```python
from build123d import *

# Parameters (mm, degrees)
F0_R     = 9.525
F0_R_2   = 63.5
F0_R_3   = 31.75
F0_R_4   = 19.05
F0_R_5   = 6.35
F1_DEPTH = 19.05
F2_DEPTH = 76.2
F3_DEPTH = 50.8
F4_DEPTH = 38.1


with BuildPart() as f1:
    # F0 (on Top) → F1 (new body)
    with BuildSketch(Plane.XY):
        with BuildLine():
            ThreePointArc((0, 76.2), (53.881537, 53.881537), (76.2, 0))
            Line((76.2, 0), (88.9, 0))
            Line((88.9, 0), (88.9, 38.1))
            Line((88.9, 38.1), (107.95, 38.1))
            ThreePointArc((107.95, 38.1), (127, 57.15), (107.95, 76.2))
            Line((107.95, 76.2), (0, 76.2))
        make_face()
        with Locations((107.95, 57.15)):
            Circle(F0_R, mode=Mode.SUBTRACT)
        with BuildLine():
            ThreePointArc((-76.2, 0), (-53.881537, 53.881537), (0, 76.2))
            Line((0, 76.2), (-107.95, 76.2))
            ThreePointArc((-107.95, 76.2), (-127, 57.15), (-107.95, 38.1))
            Line((-107.95, 38.1), (-88.9, 38.1))
            Line((-88.9, 38.1), (-88.9, 0))
            Line((-88.9, 0), (-76.2, 0))
        make_face()
        with Locations((-107.95, 57.15)):
            Circle(F0_R, mode=Mode.SUBTRACT)
        with BuildLine():
            Line((-107.95, -76.2), (0, -76.2))
            ThreePointArc((0, -76.2), (-53.881537, -53.881537), (-76.2, 0))
            Line((-76.2, 0), (-88.9, 0))
            Line((-88.9, 0), (-88.9, -38.1))
            Line((-88.9, -38.1), (-107.95, -38.1))
            ThreePointArc((-107.95, -38.1), (-127, -57.15), (-107.95, -76.2))
        make_face()
        with Locations((-107.95, -57.15)):
            Circle(F0_R, mode=Mode.SUBTRACT)
        with BuildLine():
            Line((88.9, 0), (76.2, 0))
            ThreePointArc((76.2, 0), (53.881537, -53.881537), (0, -76.2))
            Line((0, -76.2), (107.95, -76.2))
            ThreePointArc((107.95, -76.2), (127, -57.15), (107.95, -38.1))
            Line((107.95, -38.1), (88.9, -38.1))
            Line((88.9, -38.1), (88.9, 0))
        make_face()
        with Locations((107.95, -57.15)):
            Circle(F0_R, mode=Mode.SUBTRACT)
        with BuildLine():
            ThreePointArc((0, -76.2), (53.881537, -53.881537), (76.2, 0))
            ThreePointArc((76.2, 0), (53.881537, 53.881537), (0, 76.2))
            ThreePointArc((0, 76.2), (-53.881537, 53.881537), (-76.2, 0))
            ThreePointArc((-76.2, 0), (-53.881537, -53.881537), (0, -76.2))
        make_face()
        Circle(F0_R_2, mode=Mode.SUBTRACT)
        Circle(F0_R_2)
        Circle(F0_R_3, mode=Mode.SUBTRACT)
        Circle(F0_R_3)
        Circle(F0_R_4, mode=Mode.SUBTRACT)
        Circle(F0_R_4)
        Circle(F0_R_5, mode=Mode.SUBTRACT)
        Circle(F0_R_5)
    extrude(amount=F1_DEPTH)

    # F0 (on Top) → F2 (join)
    with BuildSketch(Plane.XY):
        with BuildLine():
            ThreePointArc((0, -76.2), (53.881537, -53.881537), (76.2, 0))
            ThreePointArc((76.2, 0), (53.881537, 53.881537), (0, 76.2))
            ThreePointArc((0, 76.2), (-53.881537, 53.881537), (-76.2, 0))
            ThreePointArc((-76.2, 0), (-53.881537, -53.881537), (0, -76.2))
        make_face()
        Circle(F0_R_2, mode=Mode.SUBTRACT)
    extrude(amount=F2_DEPTH)

    # F0 (on Top) → F3 (join)
    with BuildSketch(Plane.XY):
        Circle(F0_R_3)
        Circle(F0_R_4, mode=Mode.SUBTRACT)
    extrude(amount=F3_DEPTH)

    # F0 (on Top) → F4 (join)
    with BuildSketch(Plane.XY):
        Circle(F0_R_4)
        Circle(F0_R_5, mode=Mode.SUBTRACT)
    extrude(amount=F4_DEPTH)


solid = f1.part
```
CAD build for the part. Positions are in the model's coordinates, mm. A direction names the side the tool comes from. Round coordinates to 2 decimals unless told otherwise and drop trailing zeros. Write each loop counter-clockwise with the first axis right and the second up, starting at its lowest first coordinate (ties: lowest second). Pieces come first, ordered by that corner, then holes. Notation, with made-up numbers: (34, -10) - (54, -10) arc R33 ccw to (54, 26) - close; hole circle Ø10 at (-0.5, 82). An arc over 180 degrees is marked (long way). Return JSON: item names as keys, results as strings. Group by question number.
Item 1: Band-saw the part on D-D on z = 7. List the corners of the cut face in (x, y) (3 decimals).
Item 2: 3-axis set-ups, long thin cutter, end or side, ignore diameter. For faces 1 (the face through (0, 0, 19.05)), 2 (the face through (98, 38.1, 9)), 3 (the face through (-114.97, -50.71, 9.39)), 4 (the face through (-99, 38.1, 9)): which of +Z, -Z, +X, -X, +Y, -Y reach the whole face in a straight line?
Item 3: Probe probe 1 along Y at (x, z) = (-107.95, 9.75) (3 decimals); probe 2 along Y at (x, z) = (-89.5, 6.5); probe 3 along Z at (x, y) = (-74.5, -30.5). List the from-to ranges inside material, lowest first.
Item 4: Band-saw the part on B-B on y = -61. List the corners of the cut face in (x, z), plus the area to 3 significant figures.
Item 5: Band-saw the part on C-C on x = -94.5. List the corners of the cut face in (y, z), plus the area to 3 significant figures.
Item 6: Mould opens along X. For faces 5 (the face through (-5, 5, 38.1)), 6 (the face through (82, 0, 19.05)), 7 (the face through (112.35, 48.7, 9.39)), 8 (the face through (88.9, -1, 9)) say: +X half, -X half, draft (parallel to the pull), parting line (faces both ways), or undercut.
Item 7: Flat gauge pins, fed straight in: pin 1 Ø4 at (x, z) = (-28.5, 37.5) entering from -Y; pin 2 Ø25 at (x, y) = (107.95, -57.15) entering from +Z; pin 3 Ø21 at (y, z) = (3, 8) entering from +X. Where does each tip first touch, or does it go through?
Item 8: Band-saw the part on A-A on z = 47. List the corners of the cut face in (x, y).
Resolved:
{
 "1": {"outline": "(-107.95, -76.2) - (107.95, -76.2) arc R19.05 ccw to (107.95, -38.1) - (88.9, -38.1) - (88.9, 38.1) - (107.95, 38.1) arc R19.05 ccw to (107.95, 76.2) - (-107.95, 76.2) arc R19.05 ccw to (-107.95, 38.1) - (-88.9, 38.1) - (-88.9, -38.1) - (-107.95, -38.1) arc R19.05 ccw to start; hole circle Ø19.05 at (-107.95, -57.15); hole circle Ø19.05 at (-107.95, 57.15); hole circle Ø19.05 at (107.95, -57.15); hole circle Ø19.05 at (107.95, 57.15)"},
 "2": {"face 1": "+Z", "face 2": "+Z, -Z, +X", "face 3": "+Z, -Z", "face 4": "+Z, -Z, -X"},
 "3": {"probe 1": "y = -76.2 to -66.675, -47.625 to -38.1, 38.1 to 47.625, 66.675 to 76.2", "probe 2": "y = -76.2 to -38.1, 38.1 to 76.2", "probe 3": "z = 0 to 19.05"},
 "4": {"outline": "(-126.61, 0) - (-116.66, 0) - (-116.66, 19.05) - (-126.61, 19.05) - close; (-99.24, 0) - (99.24, 0) - (99.24, 19.05) - (45.67, 19.05) - (45.67, 76.2) - (17.64, 76.2) - (17.64, 19.05) - (-17.64, 19.05) - (-17.64, 76.2) - (-45.67, 76.2) - (-45.67, 19.05) - (-99.24, 19.05) - close; (116.66, 0) - (126.61, 0) - (126.61, 19.05) - (116.66, 19.05) - close", "area": "7,360 mm²"},
 "5": {"outline": "(-76.2, 0) - (-38.1, 0) - (-38.1, 19.05) - (-76.2, 19.05) - close; (38.1, 0) - (76.2, 0) - (76.2, 19.05) - (38.1, 19.05) - close", "area": "1,450 mm²"},
 "6": {"face 5": "undercut", "face 6": "draft", "face 7": "undercut", "face 8": "+X half"},
 "7": {"pin 1": "stops at y = -71.44", "pin 2": "stops at z = 19.05", "pin 3": "stops at x = 88.9"},
 "8": {"outline": "(-76.2, 0) arc R76.2 ccw to (0, -76.2) arc R76.2 ccw to (76.2, 0) arc R76.2 ccw to (0, 76.2) arc R76.2 ccw to start; circle Ø63.5 at (0, 0); hole circle Ø127 at (0, 0); hole circle Ø38.1 at (0, 0)"}
}
